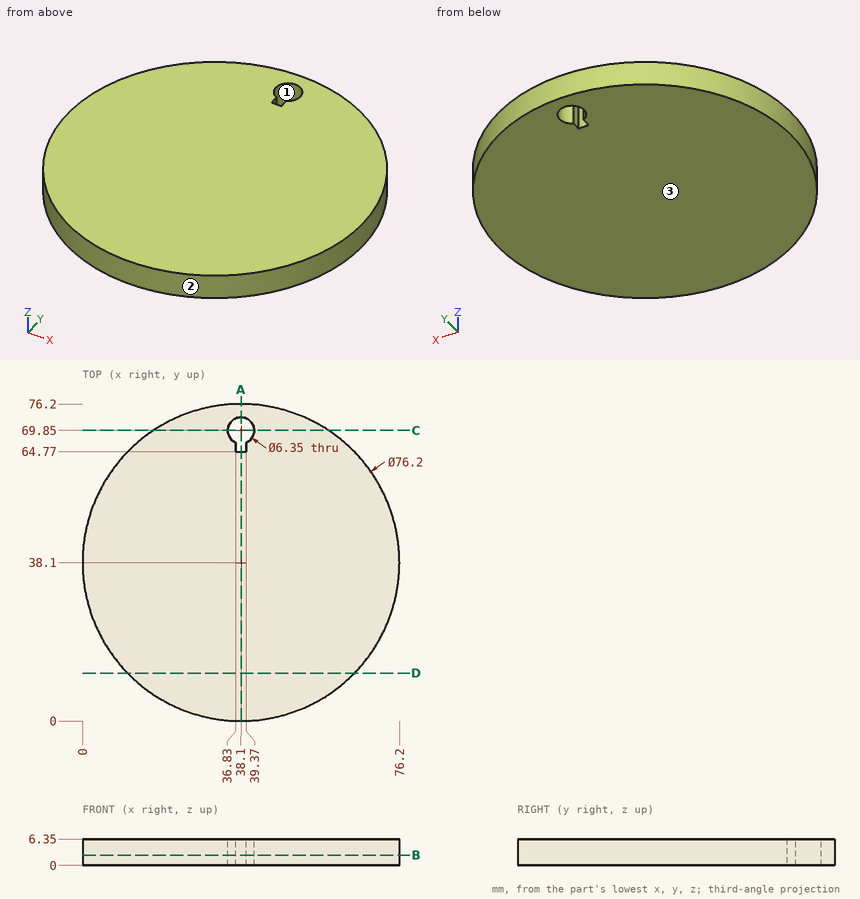
Geometry check sheet. Reference: drawing and pictorial views, mm from the part's lowest x, y, z. Give positions to 0.01 mm unless a question says otherwise; leave off trailing zeros. Write each loop counter-clockwise with the first axis right and the second up, starting at its lowest first coordinate (ties: lowest second). Pieces come first, ordered by that corner, then holes. Notation, with made-up numbers: (77, -11.75) -> (127, -11.75) arc R25 cw to (127, 24.25) -> close; hole circle Ø2 at (-22, 51). An arc over 180 degrees is marked (long way). One line per item, written item: value. Start each with the question number.
Item 1: Gauge pin test, flat ends, axial feed: pin 1 (1.7 mm diameter, centred on y = 66, z = 1.5, fed in from -X); pin 2 (3 mm diameter, centred on x = 38.5, z = 2.5, fed in from +Y); pin 3 (1.5 mm diameter, centred on x = 13, z = 5, fed in from +Y). Record the tip position at first contact, or that the pin passes through.
Item 2: Section check A-A on x = 38.1. Record the cut outline in (y, z) (3 decimals), then the cut area to 3 significant figures.
Item 3: Draft check along X on the marked faces 1, 2 and 3. Enter one of: +X half, -X half, draft (parallel to the pull), parting line (faces both ways), or undercut.
Item 4: Section check C-C on y = 69.85. Record the cut outline in (x, z) (3 decimals), then the cut area to 3 significant figures.
Item 5: Section check B-B on z = 2.5. Record the cut outline in (x, y) (3 decimals), then the cut area to 3 significant figures.
Item 6: Section check D-D on y = 11.5. Record the cut outline in (x, z), then the cut area to 3 significant figures.
Item 7: Material ranges on probe 1 along Y at (x, z) = (38.1, 1.75) (3 decimals); probe 2 along X at (y, z) = (66, 4.25); probe 3 along X at (y, z) = (71, 5), recorded low to high. Write a range as from..to.
Results list:
1. pin 1: x = 11.27
1. pin 2: y = 76.2
1. pin 3: y = 67.4
2. outline: (0, 0) -> (64.77, 0) -> (64.77, 6.35) -> (0, 6.35) -> close; (73.025, 0) -> (76.2, 0) -> (76.2, 6.35) -> (73.025, 6.35) -> close
2. area: 431 mm²
3. face 1: undercut
3. face 2: parting line
3. face 3: draft
4. outline: (17.039, 0) -> (34.925, 0) -> (34.925, 6.35) -> (17.039, 6.35) -> close; (41.275, 0) -> (59.161, 0) -> (59.161, 6.35) -> (41.275, 6.35) -> close
4. area: 227 mm²
5. outline: circle Ø76.2 at (38.1, 38.1); hole (36.83, 64.77) -> (39.37, 64.77) -> (39.37, 66.94) arc R3.175 ccw (long way) to (36.83, 66.94) -> close
5. area: 4,520 mm²
6. outline: (10.82, 0) -> (65.38, 0) -> (65.38, 6.35) -> (10.82, 6.35) -> close
6. area: 346 mm²
7. probe 1: 0..64.77, 73.025..76.2
7. probe 2: 12.15..36.83, 39.37..64.05
7. probe 3: 18.89..35.14, 41.06..57.31
